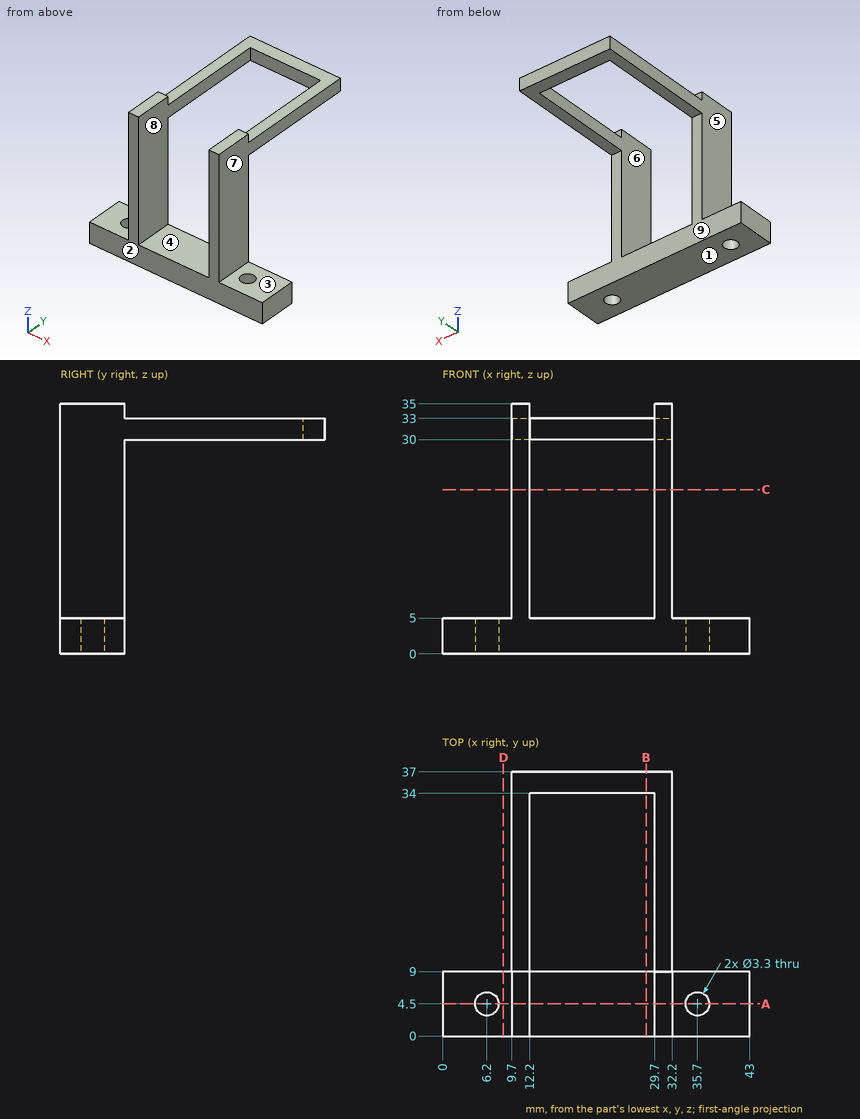
Print and shaded views of the part. All mm, measured from the part's lowest x, y and z. A direction names the side the tool comes from. Coordinates: 2 decimals unless noted, no trailing zeros. Write each loop counter-clockwise with the first axis right and the second up, starting at its lowest first coordinate (ties: lowest second). Pieces come first, ordered by that corner, then holes. Notation, with made-up numbers: M -17,72 L 38,72 A11 cw 38,93 Z; hole C 23,68 d3. An arc over 180 degrees is marked long. Return JSON: item names as keys, results as strings.
1. Saw through at B-B, the plane x = 28.5. Write the cut outline in (y, z).
Determined:
{"outline": "M 0,0 L 9,0 L 9,5 L 0,5 Z; M 34,30 L 37,30 L 37,33 L 34,33 Z"}
2. Saw through at D-D, the plane x = 8.5. Write the cut outline in (y, z), then the cut area to 3 significant figures.
Determined:
{"outline": "M 0,0 L 9,0 L 9,5 L 0,5 Z", "area": "45.0 mm²"}
3. Flat gauge pins, fed straight in: pin 1 Ø10 at (x, y) = (21, 5.5) entering from +Z; pin 2 Ø12 at (y, z) = (5.5, 10) entering from -X; pin 3 Ø3.5 at (x, z) = (24.5, 32) entering from -Y; pin 4 Ø1.5 at (x, z) = (6, 5) entering from +Y. Where does each tip first touch, or does it go through?
Determined:
{"pin 1": "z = 5", "pin 2": "x = 0", "pin 3": "y = 34", "pin 4": "y = 9"}
4. 3-axis set-ups, long thin cutter, end or side, ignore diameter. For the marked faces 1, 2, 3, 4 and 5: which of +Z, -Z, +X, -X, +Y, -Y reach the whole face in a straight line?
Determined:
{"face 1": "-Z, +X, -X, +Y, -Y", "face 2": "+Z, -Z, +X, -X, -Y", "face 3": "+Z, +X, +Y, -Y", "face 4": "+Z, +Y, -Y", "face 5": "+Z, -X, +Y, -Y"}
5. Probe L1, parallel to X at y = 4.5, z = 3.65; L2, parallel to Y at x = 6.2, z = 3.9; L3, parallel to Y at x = 27, z = 3.5. List the from-to ranges inside material, lowest first.
Determined:
{"L1": "0 to 4.55, 7.85 to 34.05, 37.35 to 43", "L2": "0 to 2.85, 6.15 to 9", "L3": "0 to 9"}
6. Saw through at A-A, the plane y = 4.5. Write the cut outline in (x, z), then the cut area to 3 significant figures.
Determined:
{"outline": "M 0,0 L 4.55,0 L 4.55,5 L 0,5 Z; M 7.85,0 L 34.05,0 L 34.05,5 L 32.2,5 L 32.2,35 L 29.7,35 L 29.7,5 L 12.2,5 L 12.2,35 L 9.7,35 L 9.7,5 L 7.85,5 Z; M 37.35,0 L 43,0 L 43,5 L 37.35,5 Z", "area": "332 mm²"}
7. Pull direction X, two halves, no side cores. Call the marked faces 6, 7, 8 and 9: pulls with the +X half, pulls with the -X half, needs draft (parallel to the pull), parting line crosses it, or undercut.
Determined:
{"face 6": "undercut", "face 7": "pulls with the +X half", "face 8": "undercut", "face 9": "needs draft"}
8. Saw through at C-C, the plane z = 23. Write the cut outline in (x, y).
Determined:
{"outline": "M 9.7,0 L 12.2,0 L 12.2,9 L 9.7,9 Z; M 29.7,0 L 32.2,0 L 32.2,9 L 29.7,9 Z"}
